from build123d import *

# Parameters (mm, degrees)
SKETCH1_R               = 10
BOSS_EXTRUDE1_DEPTH     = 276
SKETCH2_R               = 14
BOSS_EXTRUDE2_DEPTH     = 56
CUT_EXTRUDE1_DEPTH      = 56
CUT_EXTRUDE1_DEPTH_BACK = 56
SKETCH3_R               = 3.2


with BuildPart() as part:
    # Sketch1 → Boss-Extrude1 (new body)
    with BuildSketch(Plane.XY):
        Circle(SKETCH1_R)
    extrude(amount=BOSS_EXTRUDE1_DEPTH)

    # Sketch2 → Boss-Extrude2 (add)
    with BuildSketch(Plane.XY.offset(276)):
        Circle(SKETCH2_R)
    extrude(amount=-BOSS_EXTRUDE2_DEPTH)

    # Sketch3 → Cut-Extrude1 (cut, two sides: drawn at the far end of the back side and taken through both)
    with BuildSketch(Plane(origin=(0, 0, 0), x_dir=(1, 0, 0), z_dir=(0, 1, 0)).offset(-CUT_EXTRUDE1_DEPTH_BACK)):
        with Locations(Location((0, -9, 0), (0, 0, 90))):
            Circle(SKETCH3_R)
    extrude(amount=CUT_EXTRUDE1_DEPTH + CUT_EXTRUDE1_DEPTH_BACK, mode=Mode.SUBTRACT)


solid = part.part
Build history of the part. All positions in model axes, mm. A direction names the side the tool comes from. Coordinates: 2 decimals unless noted, no trailing zeros. Order: outer loops, then holes, each group sorted by start corner. A loop starts at its lowest first (then second) coordinate and runs counter-clockwise, first axis right, second up. Notation, with made-up numbers: (4, 16) - (57, 16) arc R24 cw to (57, 34) - close; hole circle Ø3 at (-8, 41). An arc over 180 degrees is marked (long way). Write each question's results on one line, items separated by ' | '. Start each with the question number.
Item 1: Band-saw the part on D-D on z = 241.5. Write the cut outline in (x, y).
Item 2: Mould opens along Z. For faces 3 (the face through (0, 0, 276)), 4 (the face through (-3, 10, 220)), 5 (the face through (1.947, -0.14, 11.539)) say: released by +Z, released by -Z, zero draft, split by the parting line, or undercut.
Item 3: Band-saw the part on C-C on z = 9. Write the cut outline in (x, y), and give its area (3 significant figures).
Item 4: Flat gauge pins, fed straight in: pin 1 (6 mm diameter, centred on y = -9, z = 156.5, fed in from -X); pin 2 (8.5 mm diameter, centred on x = 6, y = -7, fed in from -Z); pin 3 (8 mm diameter, centred on x = 5, z = 85.5, fed in from -Y); pin 4 (12 mm diameter, centred on x = 1.5, z = 60.5, fed in from +Y). Where does each tip first touch, or does it go through?
Item 5: Tool access for faces 1 (the face through (12.932, -5.362, 248.392)), 2 (the face through (9.54, 3, 108.46)): list every direction of +Z, -Z, +X, -X, +Y, -Y with a clear straight run to the whole face (end or side of a thin tool).
Item 6: Band-saw the part on B-B on y = 0. Write the cut outline in (x, z), and give its area (3 significant figures).
Item 7: Wall check: probe 1 along Z at (x, y) = (-0.5, 8.5); probe 2 along X at (y, z) = (0, 9); probe 3 along Z at (x, y) = (7, -7.75). Give the ranges that are in metal, low to high. Write a range as [from, to].
Item 8: Band-saw the part on A-A on x = 0. Write the cut outline in (y, z).
Numbers:
1) outline: circle Ø28 at (0, 0)
2) face 3: released by +Z | face 4: released by -Z | face 5: undercut
3) outline: (-3.2, -9.47) - (-3.2, 9.47) arc R10 ccw to start; (3.2, -9.47) arc R10 ccw to (3.2, 9.47) - close | area: 188 mm^2
4) pin 1: x = -8 | pin 2: z = 0 | pin 3: y = -9.95 | pin 4: y = 10
5) face 1: +Z, -Z | face 2: -Z
6) outline: (-14, 220) - (-10, 220) - (-10, 0) - (10, 0) - (10, 220) - (14, 220) - (14, 276) - (-14, 276) - close; hole circle Ø6.4 at (0, 9) | area: 5,940 mm^2
7) probe 1: [0, 5.84], [12.16, 276] | probe 2: [-10, -3.2], [3.2, 10] | probe 3: [220, 276]
8) outline: (-14, 220) - (-10, 220) - (-10, 12.2) - (10, 12.2) - (10, 220) - (14, 220) - (14, 276) - (-14, 276) - close; (-10, 0) - (10, 0) - (10, 5.8) - (-10, 5.8) - close
